CAD build for the part. Positions are in the model's coordinates, mm. A direction names the side the tool comes from. Give positions to 0.01 mm unless a question says otherwise; leave off trailing zeros. Order: outer loops, then holes, each group sorted by start corner. A loop starts at its lowest first (then second) coordinate and runs counter-clockwise, first axis right, second up.
```python
from build123d import *

# Parameters (mm, degrees)
SALIENTE_EXTRUIR1_DEPTH = 2.5
VACIADO1_T              = 0.5
CROQUIS3_R              = 5.5
CORTAR_EXTRUIR1_DEPTH   = 27.241879304
REDONDEO1_R             = 0.3


with BuildPart() as part:
    # Croquis2 → Saliente-Extruir1 (new body)
    with BuildSketch(Plane(origin=(0, 0, 0), x_dir=(1, 0, 0), z_dir=(0, 1, 0))):
        Polygon((-6.46994338, 13.677119477), (-0.219892949, 0), (-6.46994338, -13.677119477), (20.44143079, 0), align=None)
    extrude(amount=SALIENTE_EXTRUIR1_DEPTH)

    # Vaciado1
    vaciado1_openings = [part.faces().sort_by_distance(p)[0] for p in [
        (4.58386482, 2.5, 0),
    ]]
    offset(amount=VACIADO1_T, openings=vaciado1_openings, kind=Kind.INTERSECTION)

    # Croquis3 → Cortar-Extruir1 (cut, through all)
    with BuildSketch(Plane(origin=(0, 0, 0), x_dir=(1, 0, 0), z_dir=(0, 1, 0))):
        with Locations(Location((6, 0, 0), (0, 0, 270))):
            Circle(CROQUIS3_R)
    extrude(amount=-CORTAR_EXTRUIR1_DEPTH, mode=Mode.SUBTRACT)

    # Redondeo1
    redondeo1_edges = [part.edges().sort_by_distance(p)[0] for p in [
        (20.44143079, 1.25, 0),
        (-6.46994338, 1.25, -13.677119477),
        (-0.219892949, 1.25, 0),
        (-6.46994338, 1.25, 13.677119477),
        (21.545007766, 1, 0),
        (-7.519801831, 1, 14.771556106),
        (-0.769625322, 1, 0),
        (-7.519801831, 1, -14.771556106),
    ]]
    fillet(redondeo1_edges, radius=REDONDEO1_R)


solid = part.part
```
Item 1: Slice it at B-B (x = 9.75). Give the cut face in (y, z).
Item 2: Tool access for faces 4 (the face through (-3.95, 0.98, 6.96)), 5 (the face through (-3.154, 1.232, 6.421)), 6 (the face through (-0.43, 2.5, -0.07)): list every direction of +Z, -Z, +X, -X, +Y, -Y with a clear straight run to the whole face (end or side of a thin tool).
Item 3: Wall check: L1, parallel to Z at x = -1.75, y = 2; L2, parallel to Z at x = -4, y = 0.05; L3, parallel to X at y = -0.1, z = 0. Give the ranges that are in metal, low to high.
Item 4: Slice it at C-C (z = 5). Give the cut face in (x, y).
Item 5: Slice it at A-A (y = 0.9). Give the cut face in (x, z).
Item 6: Drop flat-ended pins along their axis: pin 1 Ø1 at (x, y) = (9.5, 1.5) entering from -Z; pin 2 Ø1 at (y, z) = (1, 1) entering from -X. Give the stop position or say it passes through.
Item 7: Slice it at D-D (z = 10.75). Give the cut face in (x, y).
Item 8: Two-plate mould, pull along Z, no slides. Class faces 1 (the face through (-4.039, 0.979, -7.155)), 2 (the face through (7.327, 0.979, -7.226)), 3 (the face through (6.938, 0.979, 7.424)): released by +Z, released by -Z, zero draft, split by the parting line, or undercut.
A:
1. outline: (-0.5, -5.99) - (2.5, -5.99) - (2.5, -5.43) - (0, -5.43) - (0, -4.02) - (-0.5, -4.02) - close; (-0.5, 4.02) - (0, 4.02) - (0, 5.43) - (2.5, 5.43) - (2.5, 5.99) - (-0.5, 5.99) - close
2. face 4: -X, +Y, -Y
2. face 5: +Y
2. face 6: +Z, -Z, +X, -X, +Y
3. L1: z = -11.84 to -11.28, -3.35 to -2.15, 2.15 to 3.35, 11.28 to 11.84
3. L2: z = -12.98 to -12.42, -8.27 to -7.07, 7.07 to 8.27, 12.42 to 12.98
3. L3: x = -0.8 to 0.5, 11.5 to 21.18
4. outline: (-3.05, -0.5) - (3.71, -0.5) - (3.71, 0) - (-2.5, 0) - (-2.5, 2.5) - (-3.05, 2.5) - close; (8.29, -0.5) - (11.71, -0.5) - (11.71, 2.5) - (10.6, 2.5) - (10.6, 0) - (8.29, 0) - close
5. outline: (-7.16, -13.99) arc R0.3 ccw to (-6.75, -14.38) - (21.02, -0.27) arc R0.3 ccw to (21.02, 0.27) - (-6.75, 14.38) arc R0.3 ccw to (-7.16, 13.99) - (-0.83, 0.12) arc R0.3 cw to (-0.83, -0.12) - close; hole (-6.11, -12.9) arc R0.3 ccw to (-5.7, -13.29) - (19.92, -0.27) arc R0.3 ccw to (19.92, 0.27) - (-5.7, 13.29) arc R0.3 ccw to (-6.11, 12.9) - (-0.28, 0.12) arc R0.3 cw to (-0.28, -0.12) - close
6. pin 1: stops at z = -6.38
6. pin 2: stops at x = -1.46
7. outline: (-5.68, -0.5) - (0.39, -0.5) - (0.39, 2.5) - (-0.71, 2.5) - (-0.71, 0) - (-5.13, 0) - (-5.13, 2.5) - (-5.68, 2.5) - close
8. face 1: undercut
8. face 2: released by -Z
8. face 3: released by +Z
